Part model, mm, in its own coordinate system. A direction names the side the tool comes from. Give positions to 0.01 mm unless a question says otherwise; leave off trailing zeros. Write each loop counter-clockwise with the first axis right and the second up, starting at its lowest first coordinate (ties: lowest second). Pieces come first, ordered by that corner, then holes. Notation, with made-up numbers: M -38.75,68 L -5.75,68 A28 ccw -5.75,105 Z; hole C 36.5,63.25 d4. An arc over 180 degrees is marked long. Use a Markdown table: item, result.
```python
from build123d import *
from build123d.topology import SkipClean

# Parameters (mm, degrees)
SKETCH1_R            = 5
BOSS_EXTRUDE1_DEPTH  = 8
BOSS_EXTRUDE2_START  = 28
SKETCH2_R            = 11
SKETCH2_R_2          = 5
BOSS_EXTRUDE2_DEPTH  = 28
M4_CLEARANCE_HOLE1_D = 4.5
CIRPATTERN1_COUNT    = 8
FILLET1_R            = 1
FILLET2_R            = 0.5


with BuildPart() as part:
    # Sketch1 → Boss-Extrude1 (new body)
    with BuildSketch(Plane(origin=(0, 0, 0), x_dir=(1, 0, 0), z_dir=(0, 1, 0))):
        with BuildLine():
            Line((-14.947825929, 14.75), (14.947825929, 14.75))
            ThreePointArc((14.947825929, 14.75), (21, 0), (14.947825929, -14.75))
            Line((14.947825929, -14.75), (-14.947825929, -14.75))
            ThreePointArc((-14.947825929, -14.75), (-21, 0), (-14.947825929, 14.75))
        make_face()
        with Locations(Location((0, 0, 0), (0, 0, 270))):
            Circle(SKETCH1_R, mode=Mode.SUBTRACT)
    extrude(amount=BOSS_EXTRUDE1_DEPTH)

    # Sketch2 → Boss-Extrude2 (add)
    with SkipClean():  # the faces are left unmerged after this step: merging them gives an invalid solid
        with BuildSketch(Plane.XZ.offset(BOSS_EXTRUDE2_START)):
            with Locations(Location((0, 0, 0), (0, 0, 90))):
                Circle(SKETCH2_R)
            with Locations(Location((0, 0, 0), (0, 0, 270))):
                Circle(SKETCH2_R_2, mode=Mode.SUBTRACT)
        extrude(amount=-BOSS_EXTRUDE2_DEPTH)

    # M4 Clearance Hole1 (through all)
    with Locations(Plane(origin=(0, 8, 0), x_dir=(1, 0, 0), z_dir=(0, 1, 0))):
        with Locations((16, 0)):
            m4_clearance_hole1 = Hole(M4_CLEARANCE_HOLE1_D / 2)

    # CirPattern1: M4 Clearance Hole1 ×8 about axis, 2 skipped
    with SkipClean():  # the faces are left unmerged after this step: merging them gives an invalid solid
        cirpattern1_axis = Axis((0, 0, 0), (0, 1, 0))
        add([m4_clearance_hole1.rotate(cirpattern1_axis, i * 360 / CIRPATTERN1_COUNT) for i in range(1, CIRPATTERN1_COUNT) if i not in (2, 6)], mode=Mode.SUBTRACT)

    # Fillet1
    fillet1_edges = [part.edges().sort_by_distance(p)[0] for p in [
        (21, 8, 0),
        (-21, 8, 0),
    ]]
    fillet(fillet1_edges, radius=FILLET1_R)

    # Fillet2
    fillet2_edges = [part.edges().sort_by_distance(p)[0] for p in [
        (0, -28, -11),
        (21, 0, 0),
        (-21, 0, 0),
    ]]
    fillet(fillet2_edges, radius=FILLET2_R)


solid = part.part
```
1. Cut at C-C, the plane x = 13. Give the cut face in (y, z), then the cut area to 3 significant figures.
Findings below:
| item | result |
|---|---|
| outline | M 0,-14.75 L 8,-14.75 L 8,-12.8 L 0,-12.8 Z; M 0,-9.82 L 8,-9.82 L 8,9.82 L 0,9.82 Z; M 0,12.8 L 8,12.8 L 8,14.75 L 0,14.75 Z |
| area | 188 mm2 |
2. Two-plate mould, pull along Z, no slides. Class faces 3 (the flat face through (-4.2, 8, 3.1)), 4 (the cylindrical face through (-21, 4, 0)), 5 (the cylindrical face through (11.41, 3.94, -13.56)): released by +Z, released by -Z, zero draft, split by the parting line, or undercut.
Findings below:
| item | result |
|---|---|
| face 3 | zero draft |
| face 4 | split by the parting line |
| face 5 | undercut |
3. Cut at A-A, the plane x = 0. Give the cut face in (y, z).
Findings below:
| item | result |
|---|---|
| outline | M -28,-10.5 A0.5 ccw -27.5,-11 L 0,-11 L 0,-14.75 L 8,-14.75 L 8,-5 L -28,-5 Z; M -28,5 L 8,5 L 8,14.75 L 0,14.75 L 0,11 L -27.5,11 A0.5 ccw -28,10.5 Z |
4. Drill centre lines: L1, parallel to Y at x = 1, z = -11.25; L2, parallel to X at y = 2.5, z = 11; L3, parallel to X at y = -23, z = -2.75. Where is each one in solid material? Low to high.
Findings below:
| item | result |
|---|---|
| L1 | 0 to 8 |
| L2 | -17.89 to -13.54, -9.09 to 9.09, 13.54 to 17.89 |
| L3 | -10.65 to -4.18, 4.18 to 10.65 |
5. Cut at D-D, the plane y = -8. Give the cut face in (x, z).
Findings below:
| item | result |
|---|---|
| outline | C 0,0 d22; hole C 0,0 d10 |
6. Cut at B-B, the plane z = 0. Give the cut face in (x, y), then the cut area to 3 significant figures.
Findings below:
| item | result |
|---|---|
| outline | M -21,0.5 A0.5 ccw -20.5,0 L -18.25,0 L -18.25,8 L -20,8 A1 ccw -21,7 Z; M -13.75,0 L -11,0 L -11,-27.5 A0.5 ccw -10.5,-28 L -5,-28 L -5,8 L -13.75,8 Z; M 5,-28 L 10.5,-28 A0.5 ccw 11,-27.5 L 11,0 L 13.75,0 L 13.75,8 L 5,8 Z; M 18.25,0 L 20.5,0 A0.5 ccw 21,0.5 L 21,7 A1 ccw 20,8 L 18.25,8 Z |
| area | 519 mm2 |
7. Tool access for faces 1 (the flat face through (0, 4, 14.75)), 2 (the flat face through (5, 0, -10)): list every direction of +Z, -Z, +X, -X, +Y, -Y with a clear straight run to the whole face (end or side of a thin tool).
Findings below:
| item | result |
|---|---|
| face 1 | +Z, +X, -X, +Y, -Y |
| face 2 | -Y |
8. Drop flat-ended pins along their axis: P1, Ø6, axis at x = -16.5, z = -9, coming from the -Y side; P2, Ø3, axis at x = -3.5, y = -2, coming from the -Z side; P3, Ø3, axis at y = -16, z = -4, coming from the +X side. Give the stop position or say it passes through.
Findings below:
| item | result |
|---|---|
| P1 | y = 0 |
| P2 | z = -10.82 |
| P3 | x = 10.71 |
